Study the drawing (mm; zero at the part's minimum x, y, z) and answer. A direction names the side the tool comes from. Coordinates: 2 decimals unless noted, no trailing zeros. Loops run counter-clockwise (first coordinate to the right, second up) from the corner with the lowest first, then second, coordinate; pieces in that order, holes last. Notation, with made-up numbers: (28.25, -19) - (81.25, -19) arc R27 ccw to (81.25, 15) - close; hole circle Ø8 at (89, 52). An arc over 180 degrees is marked (long way). Write each question's results on one line, items separated by ' | '. Start each with the question number.
(1) Given pin 1 Ø5.5 at (x, y) = (4, 6) entering from +Z; pin 2 Ø2 at (x, z) = (1.5, 8.5) entering from -Y; pin 3 Ø3 at (x, z) = (38, 3) entering from -Y, each flat-ended and moving along its own axis, determine where each tip first touches the part or whether it passes through.
(2) For the marked faces 1 and 2, determine the directions among +Z, -Z, +X, -X, +Y, -Y from which every point of the face is accessible in a straight line to the end or side of a thin tool.
(3) Find section C-C on x = 98. Determine the outline of the cut face in (y, z), then the cut area to 3 significant figures.
(4) Find section B-B on y = 19.5. Determine the outline of the cut face in (x, z), then the cut area to 3 significant figures.
(5) Consider line 1 (X direction, y = 33.4, z = 5); line 2 (X direction, y = 25.5, z = 5.5); line 3 (Z direction, x = 98, y = 33.9). Determine where each line is inside the solid, lowest interval first. Write a range as from..to.
(6) Find section D-D on x = 44.5. Determine the outline of the cut face in (y, z), then the cut area to 3 significant figures.
(7) Find section A-A on z = 3.5. Determine the outline of the cut face in (x, y).
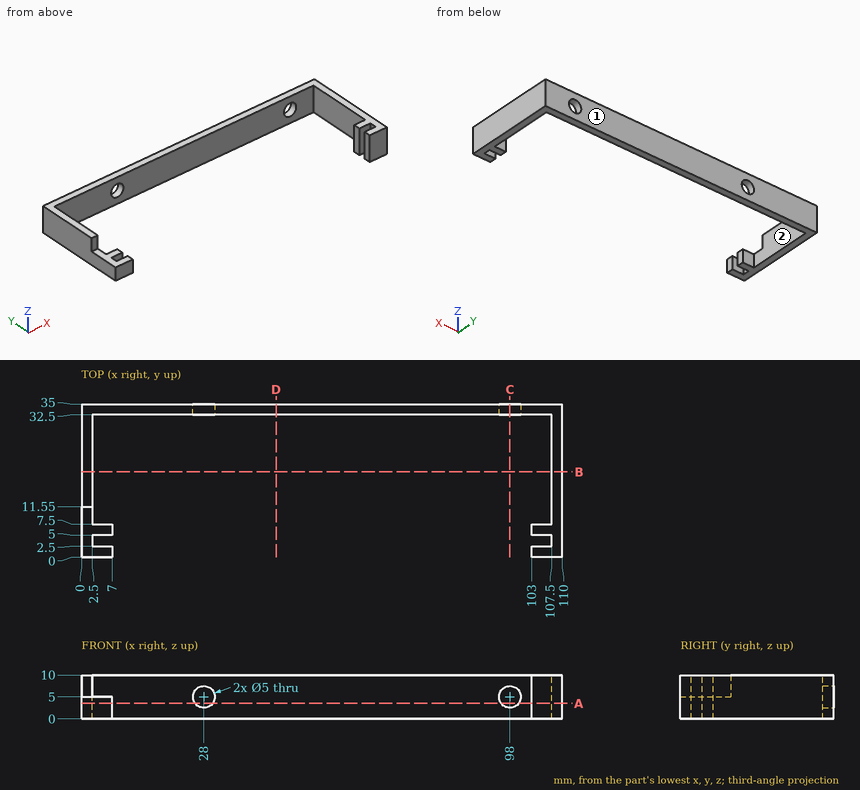
Values:
1) pin 1: stops at z = 5 | pin 2: stops at y = 11.55 | pin 3: stops at y = 32.5
2) face 1: +Z, -Z, +X, -X, +Y | face 2: +Z, -Z
3) outline: (32.5, 0) - (35, 0) - (35, 2.5) - (32.5, 2.5) - close; (32.5, 7.5) - (35, 7.5) - (35, 10) - (32.5, 10) - close | area: 12.5 mm²
4) outline: (0, 0) - (2.5, 0) - (2.5, 10) - (0, 10) - close; (107.5, 0) - (110, 0) - (110, 10) - (107.5, 10) - close | area: 50.0 mm²
5) line 1: x = 0..25.5, 30.5..95.5, 100.5..110 | line 2: x = 0..2.5, 107.5..110 | line 3: z = 0..2.5, 7.5..10
6) outline: (32.5, 0) - (35, 0) - (35, 10) - (32.5, 10) - close | area: 25.0 mm²
7) outline: (0, 0) - (7, 0) - (7, 2.5) - (2.5, 2.5) - (2.5, 5) - (7, 5) - (7, 7.5) - (2.5, 7.5) - (2.5, 32.5) - (26, 32.5) - (26, 35) - (0, 35) - close; (30, 32.5) - (96, 32.5) - (96, 35) - (30, 35) - close; (100, 32.5) - (107.5, 32.5) - (107.5, 7.5) - (103, 7.5) - (103, 5) - (107.5, 5) - (107.5, 2.5) - (103, 2.5) - (103, 0) - (110, 0) - (110, 35) - (100, 35) - close
